Job drawing, mm, ordinate dimensions from the low corner. One solid piece. Round coordinates to 2 decimals unless told otherwise and drop trailing zeros. Loops run counter-clockwise (first coordinate to the right, second up) from the corner with the lowest first, then second, coordinate; pieces in that order, holes last. Notation, with made-up numbers: M -38.75,62.5 L 10.25,62.5 A9 cw 10.25,69.5 Z; hole C -29,62.25 d1. An arc over 180 degrees is marked long. One line per item, written item: value.
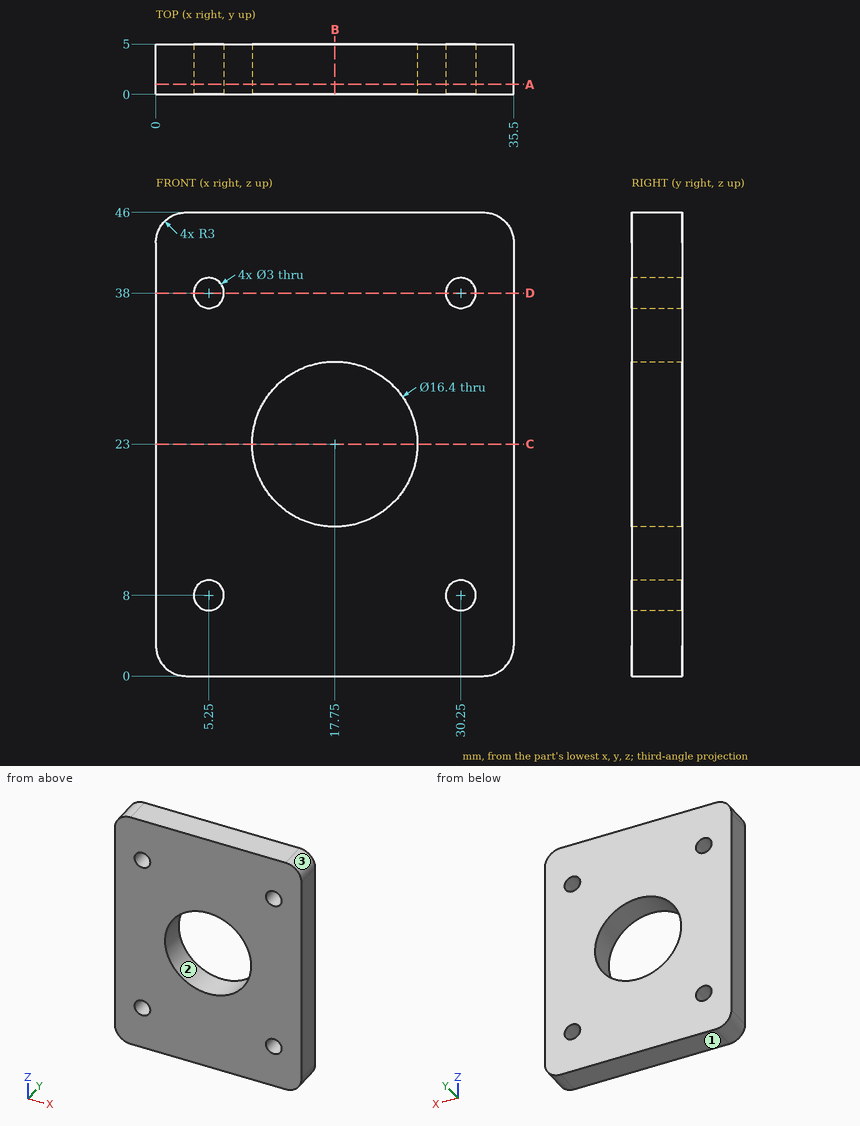
Item 1: Slice it at D-D, the plane z = 38. Give the cut face in (x, y), and give its area (4 significant figures).
Check values:
outline: M 0,0 L 3.75,0 L 3.75,5 L 0,5 Z; M 6.75,0 L 28.75,0 L 28.75,5 L 6.75,5 Z; M 31.75,0 L 35.5,0 L 35.5,5 L 31.75,5 Z
area: 147.5 mm2
Item 2: Wall check: line 1 along X through (y, z) = (3, 8); line 2 along Z through (x, y) = (18, 0.3); line 3 along X through (y, z) = (3.1, 21). Give the ranges that are in metal, low to high.
Check values:
line 1: x = 0 to 3.75, 6.75 to 28.75, 31.75 to 35.5
line 2: z = 0 to 14.8, 31.2 to 46
line 3: x = 0 to 9.8, 25.7 to 35.5
Item 3: Slice it at B-B, the plane x = 17.75. Give the cut face in (y, z).
Check values:
outline: M 0,0 L 5,0 L 5,14.8 L 0,14.8 Z; M 0,31.2 L 5,31.2 L 5,46 L 0,46 Z
Item 4: Pull direction X, two halves, no side cores. Call the marked faces 1, 2 and 3: pulls with the +X half, pulls with the -X half, needs draft (parallel to the pull), parting line crosses it, or undercut.
Check values:
face 1: needs draft
face 2: undercut
face 3: pulls with the +X half
Item 5: Slice it at C-C, the plane z = 23. Give the cut face in (x, y), and give its area (3 significant figures).
Check values:
outline: M 0,0 L 9.55,0 L 9.55,5 L 0,5 Z; M 25.95,0 L 35.5,0 L 35.5,5 L 25.95,5 Z
area: 95.5 mm2
Item 6: Drop a flat-ended pin along its axis: P1, Ø5, axis at x = 30.25, z = 38, coming from the -Y side. Give the stop position or say it passes through.
Check values:
P1: stops at y = 0
Item 7: Slice it at A-A, the plane y = 1. Give the cut face in (x, z).
Check values:
outline: M 0,3 A3 ccw 3,0 L 32.5,0 A3 ccw 35.5,3 L 35.5,43 A3 ccw 32.5,46 L 3,46 A3 ccw 0,43 Z; hole C 5.25,8 d3; hole C 5.25,38 d3; hole C 17.75,23 d16.4; hole C 30.25,8 d3; hole C 30.25,38 d3
